The listing builds one solid part. Answer for the finished solid, in the listing's coordinates (mm). A direction names the side the tool comes from. Round coordinates to 2 decimals unless told otherwise and drop trailing zeros. Write each loop counter-clockwise with the first axis right and the second up, starting at its lowest first coordinate (ties: lowest second). Pieces come first, ordered by that corner, then holes.
(1) The mould has two halves that part along Y. Classify faces 5 (the face through (0.986, 14.239, -57.765)), 6 (the face through (1, 2.5, -4.5)), 7 (the face through (0.99, 22.13, -19)), 8 (the face through (1, 8.7, 3)): +Y half, -Y half, draft (parallel to the pull), parting line (faces both ways), or undercut.
(2) Each of these flat-tipped pins is pushed along its axis until it touches: pin 1 Ø1 at (x, z) = (1, -49.5) entering from +Y; pin 2 Ø0.6 at (x, z) = (1, 3.5) entering from -Y. Where does it stop, or does it pass through?
(3) A cutting plane is placed at A-A, the plane y = 18.5. Give the vertices of the cut face in (x, z), and give its area (3 significant figures).
(4) For faces 1 (the face through (1, 19.389, -49)), 2 (the face through (1, 12.7, 3)), 3 (the face through (0, 12, -33)), 4 (the face through (0.986, 15.831, -49.704)), determine the directions among +Z, -Z, +X, -X, +Y, -Y from which every point of the face is accessible in a straight line to the end or side of a thin tool.
(5) A cutting plane is placed at D-D, the plane z = -24.5. Give the vertices of the cut face in (x, y).
(6) A cutting plane is placed at B-B, the plane x = 0.45. Give the vertices of the cut face in (y, z), and give its area (3 significant figures).
(7) A cutting plane is placed at C-C, the plane z = -40.5. Give the vertices of the cut face in (x, y).
(8) Find the intervals of material crossed by probe 1 along Z at (x, y) = (1.35, 11.25); probe 2 along Z at (x, y) = (1.6, 2.25); probe 3 along Z at (x, y) = (1.1, 2.75), in increasing order.
from build123d import *

# Parameters (mm, degrees)
RESSALTO_EXTRUS_O1_DEPTH = 2


with BuildPart() as part:
    # Esboço1 → Ressalto-extrusão1 (new body)
    with BuildSketch(Plane(origin=(0, 0, 0), x_dir=(0, 0, -1), z_dir=(1, 0, 0))):
        with BuildLine():
            Line((47.891048788, 19.389179081), (51.568608211, 12.171562323))
            ThreePointArc((51.568608211, 12.171562323), (50.694576162, 9.481568275), (48.004582114, 10.355600324))
            Line((48.004582114, 10.355600324), (45.23762298, 15.786063389))
            ThreePointArc((45.23762298, 15.786063389), (44.888153026, 16.27331816), (44.409608959, 16.634624175))
            ThreePointArc((44.409608959, 16.634624175), (18.624536688, 22.101585643), (-6, 12.7))
            Line((-6, 12.7), (-0.449608018, 12.7))
            ThreePointArc((-0.449608018, 12.7), (1.550391982, 10.7), (-0.449608018, 8.7))
            Line((-0.449608018, 8.7), (-5.446373062, 8.7))
            ThreePointArc((-5.446373062, 8.7), (-6.646208959, 8.062107753), (-6.788438162, 6.710707165))
            ThreePointArc((-6.788438162, 6.710707165), (-2.477663677, 2.236636341), (3.730763917, 2.001023917))
            ThreePointArc((3.730763917, 2.001023917), (4.55104613, 2.557847644), (5.001705215, 3.440922931))
            ThreePointArc((5.001705215, 3.440922931), (23.834938964, 15.61229456), (36.341556093, -3))
            ThreePointArc((36.341556093, -3), (37.451213604, -5.17490134), (39.837074711, -4.656054149))
            Line((39.837074711, -4.656054149), (41.277742045, -2.945943733))
            ThreePointArc((41.277742045, -2.945943733), (49.179258899, 0.290862483), (55.956453975, 5.485139138))
            ThreePointArc((55.956453975, 5.485139138), (57.714709062, 14.363124933), (50.18816454, 19.389179081))
            Line((50.18816454, 19.389179081), (47.891048788, 19.389179081))
        make_face()
    extrude(amount=RESSALTO_EXTRUS_O1_DEPTH)


solid = part.part
Solutions:
1. face 5: parting line
1. face 6: -Y half
1. face 7: +Y half
1. face 8: undercut
2. pin 1: stops at y = 19.39
2. pin 2: stops at y = 2.6
3. outline: (0, -53.89) - (2, -53.89) - (2, -48.34) - (0, -48.34) - close; (0, -40.54) - (2, -40.54) - (2, -3.95) - (0, -3.95) - close
3. area: 84.3 mm2
4. face 1: -Z, +X, -X, +Y
4. face 2: +Z, +X, -X
4. face 3: +Z, -Z, -X, +Y, -Y
4. face 4: +X, -X
5. outline: (0, 15.46) - (2, 15.46) - (2, 22.19) - (0, 22.19) - close
6. outline: (-4.66, -39.84) - (-2.95, -41.28) arc R32.3 ccw to (5.49, -55.96) arc R8.15 ccw to (19.39, -50.19) - (19.39, -47.89) - (12.17, -51.57) arc R2 cw to (10.36, -48) - (15.79, -45.24) arc R1.99 ccw to (16.63, -44.41) arc R46.58 ccw to (12.7, 6) - (12.7, 0.45) arc R2 cw to (8.7, 0.45) - (8.7, 5.45) arc R1.45 ccw to (6.71, 6.79) arc R8.31 ccw to (2, -3.73) arc R1.99 ccw to (3.44, -5) arc R16 cw to (-3, -36.34) arc R2 ccw to start
6. area: 756 mm2
7. outline: (0, -3.87) - (2, -3.87) - (2, 18.52) - (0, 18.52) - close
8. probe 1: z = -58.34 to -51.79, -47.55 to -31.93, -9.3 to -1.47
8. probe 2: z = -52.19 to -36.45, -4.21 to 2.51
8. probe 3: z = -52.85 to -36.37, -4.7 to 3.45
